```python
from build123d import *

# Parameters (mm, degrees)
SKETCH1_R           = 31.75
SKETCH1_R_2         = 1.905
BOSS_EXTRUDE1_DEPTH = 2.54
SKETCH2_R           = 31.75
SKETCH2_R_2         = 29.21
BOSS_EXTRUDE2_DEPTH = 2.54
SKETCH3_R           = 31.75
BOSS_EXTRUDE3_DEPTH = 12.7
BOSS_EXTRUDE3_DRAFT = -50
SKETCH4_R           = 46.885270626
BOSS_EXTRUDE4_DEPTH = 2.54
BOSS_EXTRUDE5_START = -1.27
BOSS_EXTRUDE5_DEPTH = 1.524
CIRPATTERN1_COUNT   = 20


with BuildPart() as part:
    # Sketch1 → Boss-Extrude1 (new body)
    with BuildSketch(Plane(origin=(0, 0, 0), x_dir=(1, 0, 0), z_dir=(0, 1, 0))):
        with Locations(Location((0, 0, 0), (0, 0, 270))):
            Circle(SKETCH1_R)
        with Locations(Location((0, 20.574, 0), (0, 0, 270))):
            Circle(SKETCH1_R_2, mode=Mode.SUBTRACT)
        with Locations(Location((20.574, 0, 0), (0, 0, 270))):
            Circle(SKETCH1_R_2, mode=Mode.SUBTRACT)
        with Locations(Location((0, -20.574, 0), (0, 0, 270))):
            Circle(SKETCH1_R_2, mode=Mode.SUBTRACT)
        with Locations(Location((-20.574, 0, 0), (0, 0, 270))):
            Circle(SKETCH1_R_2, mode=Mode.SUBTRACT)
        with Locations(Location((0, 0, 0), (0, 0, 270))):
            Circle(SKETCH1_R_2, mode=Mode.SUBTRACT)
    extrude(amount=BOSS_EXTRUDE1_DEPTH)

    # Sketch2 → Boss-Extrude2 (add)
    with BuildSketch(Plane(origin=(0, 2.54, 0), x_dir=(1, 0, 0), z_dir=(0, 1, 0))):
        with Locations(Location((0, 0, 0), (0, 0, 270))):
            Circle(SKETCH2_R)
        with Locations(Location((0, 0, 0), (0, 0, 270))):
            Circle(SKETCH2_R_2, mode=Mode.SUBTRACT)
    extrude(amount=BOSS_EXTRUDE2_DEPTH)


with BuildPart() as boss_extrude3_tool:
    # Sketch3 → Boss-Extrude3 (with draft: the straight prism first)
    with BuildSketch(Plane.XZ):
        with Locations(Location((0, 0, 0), (0, 0, 270))):
            Circle(SKETCH3_R)
    extrude(amount=BOSS_EXTRUDE3_DEPTH)
    # Boss-Extrude3: the draft: its side faces are tilted about the plane it starts from
    boss_extrude3_sides = [boss_extrude3_tool.faces().sort_by_distance(p)[0] for p in [
        (0, -6.35, 31.75),
    ]]
    draft(boss_extrude3_sides, Plane.XZ, BOSS_EXTRUDE3_DRAFT)


with BuildPart() as part_1:
    add(part.part)

    # Boss-Extrude3: add boss_extrude3_tool
    add(boss_extrude3_tool.part)

    # Sketch4 → Boss-Extrude4 (add)
    with BuildSketch(Plane.XZ.offset(12.7)):
        with Locations(Location((0, 0, 0), (0, 0, 270))):
            Circle(SKETCH4_R)
    extrude(amount=BOSS_EXTRUDE4_DEPTH)

    # Sketch6 → Boss-Extrude5 (add)
    with BuildSketch(Plane(origin=(-39.317635313, -6.35, 0), x_dir=(0.7660444431189796, 0.6427876096865376, 0), z_dir=(-0.6427876096865376, 0.7660444431189797, 0)).offset(BOSS_EXTRUDE5_START)):
        Polygon((-7.497749953, 0), (0, -4.776593518), (7.497749953, 0), (0, 4.776593518), align=None)
    boss_extrude5 = extrude(amount=BOSS_EXTRUDE5_DEPTH)

    # CirPattern1: Boss-Extrude5 ×20 about axis
    cirpattern1_axis = Axis((0, 0, 0), (0, 1, 0))
    for i in range(1, CIRPATTERN1_COUNT):
        add(boss_extrude5.rotate(cirpattern1_axis, i * 360 / CIRPATTERN1_COUNT))


solid = part_1.part
```
Can you work these out from the model? Positions are in its coordinate system, mm. A direction names the side the tool comes from. Coordinates: 2 decimals unless noted, no trailing zeros. Answer as CSV lines item,"result".
Item 1: On a 3-axis mill with a long thin cutter (end or side, diameter ignored), from which of +Z, -Z, +X, -X, +Y, -Y can I reach the whole of each face in a straight line? I mean faces 1 (the flat face through (-19.47, -4.38, -31.71)), 2 (the flat face through (8.72, -4.38, 36.17)), 3 (the flat face through (-28.34, -4.45, 24.24)), 4 (the flat face through (14.296, -4.448, 34.444)). Say none if no direction works.
Geometry results:
face 1,"-Z, +Y"
face 2,"+Y"
face 3,"+Z, +Y"
face 4,"+X, +Y"
Item 2: I'm going to push flat-ended pins straight in: P1, Ø5, axis at x = 11, z = -21, coming from the +Y side; P2, Ø2, axis at y = -12, z = -36.5, coming from the +X side; P3, Ø2, axis at x = -23, y = 0.5, coming from the -Z side. Where does each tip first touch, or does it pass through?
Geometry results:
P1,"stops at y = 2.54"
P2,"stops at x = 30.29"
P3,"stops at z = -23.02"
Item 3: Please list where these lines run through material, in increasing order: line 1 along X through (y, z) = (1.35, 0) (3 decimals); line 2 along Y through (x, z) = (5, -26); line 3 along X through (y, z) = (4, -7).
Geometry results:
line 1,"x = -31.75 to -22.479, -18.669 to -1.905, 1.905 to 18.669, 22.479 to 31.75"
line 2,"y = -15.24 to 2.54"
line 3,"x = -30.97 to -28.36, 28.36 to 30.97"
